```python
from build123d import *

# Parameters (mm, degrees)
SKETCH4_W           = 100
SKETCH4_H           = 60
BOSS_EXTRUDE2_DEPTH = 100
CUT_EXTRUDE1_DEPTH  = 100
SKETCH7_W           = 30
SKETCH7_H           = 20
CUT_EXTRUDE2_DEPTH  = 100
SKETCH10_W          = 90
SKETCH10_H          = 50
CUT_EXTRUDE6_DEPTH  = 20
BOSS_EXTRUDE3_REACH = 89.321
BOSS_EXTRUDE4_REACH = 89.321
SKETCH13_R          = 1.5
CUT_EXTRUDE7_DEPTH  = 40
SKETCH14_W          = 20
SKETCH14_H          = 40
CUT_EXTRUDE8_DEPTH  = 10
SKETCH15_R          = 1.5
CUT_EXTRUDE9_DEPTH  = 40
SKETCH16_W          = 20
SKETCH16_H          = 40
CUT_EXTRUDE10_DEPTH = 10
SKETCH17_W          = 10
SKETCH17_H          = 20
CUT_EXTRUDE11_DEPTH = 145.568322948


with BuildPart() as part:
    # Sketch4 → Boss-Extrude2 (new body)
    with BuildSketch(Plane.XY):
        Rectangle(SKETCH4_W, SKETCH4_H)
    extrude(amount=BOSS_EXTRUDE2_DEPTH)

    # Sketch6 → Cut-Extrude1 (cut)
    with BuildSketch(Plane.XY.offset(100)):
        with BuildLine():
            Line((-10, 10), (10, 10))
            Line((10, 10), (10, 0))
            ThreePointArc((10, 0), (0, -10), (-10, 0))
            Line((-10, 0), (-10, 10))
        make_face()
    extrude(amount=-CUT_EXTRUDE1_DEPTH, mode=Mode.SUBTRACT)

    # Sketch7 → Cut-Extrude2 (cut)
    with BuildSketch(Plane(origin=(50, 0, 0), x_dir=(0, 0, -1), z_dir=(1, 0, 0))):
        with Locations((-15, 20)):
            Rectangle(SKETCH7_W, SKETCH7_H)
    extrude(amount=-CUT_EXTRUDE2_DEPTH, mode=Mode.SUBTRACT)

    # Sketch10 → Cut-Extrude6 (cut)
    with BuildSketch(Plane(origin=(0, 30, 0), x_dir=(1, 0, 0), z_dir=(0, 1, 0))):
        with Locations((0, -60)):
            Rectangle(SKETCH10_W, SKETCH10_H)
    extrude(amount=-CUT_EXTRUDE6_DEPTH, mode=Mode.SUBTRACT)

    # Sketch11 → Boss-Extrude3 (add, up to next)
    with BuildSketch(Plane.XY.offset(35), mode=Mode.PRIVATE) as boss_extrude3_sk1:
        Polygon((-45, 30), (-45, 10), (-10, 10), align=None)
    boss_extrude3_tool1 = extrude(boss_extrude3_sk1.sketch, amount=BOSS_EXTRUDE3_REACH, mode=Mode.PRIVATE) - part.part
    add(boss_extrude3_tool1.solids().sort_by_distance((-33.333333, 16.666667, 35))[0])

    # Sketch12 → Boss-Extrude4 (add, up to next)
    with BuildSketch(Plane.XY.offset(35), mode=Mode.PRIVATE) as boss_extrude4_sk1:
        Polygon((10, 10), (45, 30), (45, 10), align=None)
    boss_extrude4_tool1 = extrude(boss_extrude4_sk1.sketch, amount=BOSS_EXTRUDE4_REACH, mode=Mode.PRIVATE) - part.part
    add(boss_extrude4_tool1.solids().sort_by_distance((33.333333, 16.666667, 35))[0])

    # Sketch13 → Cut-Extrude7 (cut)
    with BuildSketch(Plane.XY.offset(100)):
        with Locations((-16.5, -25)):
            Circle(SKETCH13_R)
        with Locations((16.5, -25)):
            Circle(SKETCH13_R)
    extrude(amount=-CUT_EXTRUDE7_DEPTH, mode=Mode.SUBTRACT)

    # Sketch14 → Cut-Extrude8 (cut)
    with BuildSketch(Plane.XZ.offset(30)):
        with Locations((-16.5, 75)):
            Rectangle(SKETCH14_W, SKETCH14_H)
        with Locations((16.5, 75)):
            Rectangle(SKETCH14_W, SKETCH14_H)
    extrude(amount=-CUT_EXTRUDE8_DEPTH, mode=Mode.SUBTRACT)

    # Sketch15 → Cut-Extrude9 (cut)
    with BuildSketch(Plane(origin=(0, 0, 0), x_dir=(-1, 0, 0), z_dir=(0, 0, -1))):
        with Locations((-25, -25)):
            Circle(SKETCH15_R)
        with Locations((25, -25)):
            Circle(SKETCH15_R)
    extrude(amount=-CUT_EXTRUDE9_DEPTH, mode=Mode.SUBTRACT)

    # Sketch16 → Cut-Extrude10 (cut)
    with BuildSketch(Plane(origin=(0, -30, 0), x_dir=(-1, 0, 0), z_dir=(0, -1, 0))):
        with Locations((-25, -25)):
            Rectangle(SKETCH16_W, SKETCH16_H)
        with Locations((25, -25)):
            Rectangle(SKETCH16_W, SKETCH16_H)
    extrude(amount=-CUT_EXTRUDE10_DEPTH, mode=Mode.SUBTRACT)

    # Sketch17 → Cut-Extrude11 (cut, through all)
    with BuildSketch(Plane(origin=(50, 0, 0), x_dir=(0, 0, -1), z_dir=(1, 0, 0))):
        with Locations((-95, 20)):
            Rectangle(SKETCH17_W, SKETCH17_H)
    extrude(amount=-CUT_EXTRUDE11_DEPTH, mode=Mode.SUBTRACT)


solid = part.part
```
Source: CAD feature listing. Evaluate the final solid. Frame: model axes, mm. A direction names the side the tool comes from. Round coordinates to 2 decimals unless told otherwise and drop trailing zeros. Loops run counter-clockwise (first coordinate to the right, second up) from the corner with the lowest first, then second, coordinate; pieces in that order, holes last. Notation, with made-up numbers: M 50,-39.75 L 63,-39.75 A20 cw 63,-32.75 Z; hole C 72,10 d3. An arc over 180 degrees is marked long. Use a Markdown table: item, result. Add a question column.
1. Section query C-C on y = 26. Return the cut outline in (x, z), then the cut area to 3 significant figures.
2. Section query A-A on y = 4. Return the cut outline in (x, z), then the cut area to 3 significant figures.
3. Mould query, pull axis Z, two halves, no side actions, for faces 5 (the flat face through (-30, 10, 95)), 6 (the flat face through (-17, -25, 55)), 7 (the flat face through (1, 20, 30)). Classes: pulls with the +Z half, pulls with the -Z half, needs draft (parallel to the pull), parting line crosses it, or undercut.
4. Contact query for flat-ended pins moving along their axis: P1, Ø16, axis at x = 17, z = 77, coming from the -Y side; P2, Ø2.5, axis at x = -25, y = -25, coming from the -Z side; P3, Ø6, axis at x = 1.5, z = 51, coming from the +Y side. Output: stop coordinate, or through.
5. Section query B-B on x = -25. Return the cut outline in (y, z).
6. Line query: line 1 (Z direction, x = 16, y = -22.5); line 2 (Y direction, x = -25, z = 3); line 3 (X direction, y = 2.5, z = 9). Output: solid intervals per line, ascending.
7. Reachability of faces 1 (the cylindrical face through (-17.61, -23.99, 97.54)), 2 (the cylindrical face through (26.11, -23.99, 2.46)), 3 (the flat face through (16, -20, 75)), 4 (the flat face through (1, 20, 90)) from +Z, -Z, +X, -X, +Y, -Y: full face, straight path, thin tool, end or side. Return the list, or none.
8. Section query D-D on z = 20. Return the cut outline in (x, y).
Reported:
| question | item | result |
|---|---|---|
| 1 | outline | M -50,30 L 50,30 L 50,90 L -50,90 Z; hole M -38,35 L 38,35 L 38,85 L -38,85 Z |
| 1 | area | 2,200 mm² |
| 2 | outline | M -50,0 L -10,0 L -10,100 L -50,100 Z; M 10,0 L 50,0 L 50,100 L 10,100 Z |
| 2 | area | 8,000 mm² |
| 3 | face 5 | needs draft |
| 3 | face 6 | undercut |
| 3 | face 7 | pulls with the -Z half |
| 4 | P1 | stops at y = -20 |
| 4 | P2 | stops at z = 45 |
| 4 | P3 | stops at y = -8.93 |
| 5 | outline | M -30,0 L -26.5,0 L -26.5,5 L -30,5 Z; M -30,45 L -20,45 L -20,5 L -23.5,5 L -23.5,0 L 10,0 L 10,30 L 30,30 L 30,35 L 18.57,35 L 18.57,85 L 30,85 L 30,90 L 10,90 L 10,100 L -30,100 L -30,95 L -20,95 L -20,55 L -30,55 Z |
| 6 | line 1 | z = 0 to 5, 45 to 55, 95 to 100 |
| 6 | line 2 | y = -30 to -26.5, -23.5 to 10 |
| 6 | line 3 | x = -50 to -10, 10 to 50 |
| 7 | face 1 | +Z |
| 7 | face 2 | -Z |
| 7 | face 3 | -Y |
| 7 | face 4 | +Z, +X, -X, +Y |
| 8 | outline | M -50,-30 L -35,-30 L -35,-20 L -15,-20 L -15,-30 L 15,-30 L 15,-20 L 35,-20 L 35,-30 L 50,-30 L 50,10 L 10,10 L 10,0 A10 cw -10,0 L -10,10 L -50,10 Z |
